Solid Edge part; units mm, degrees
sketch "Sketch1" plane through (0, 0, 0) normal (0, -1, 0) x (1, 0, 0)
  arc A0 (0, 36) -> (-22.6274, 28) centre (0, 0) ccw
  line L0 (-43, 28) -> (-22.6274, 28)
  line L1 (-43, 18) -> (-43, 28)
  line L2 (-22, 18) -> (-43, 18)
  line L3 (-22, 6) -> (-22, 18)
  line L4 (-18.0278, 6) -> (-22, 6)
  arc A1 (0, 19) -> (-18.0278, 6) centre (0, 0) ccw
  arc A2 (0, 19) -> (18.0278, 6) centre (0, 0) cw
  line L5 (18.0278, 6) -> (22, 6)
  line L6 (22, 6) -> (22, 18)
  line L7 (22, 18) -> (43, 18)
  line L8 (43, 18) -> (43, 28)
  line L9 (43, 28) -> (22.6274, 28)
  arc A3 (0, 36) -> (22.6274, 28) centre (0, 0) cw
extrude "Protrusion1" add sketch "Sketch1" along normal mid plane 36
sketch "Sketch2" plane through (32.8137, 0, 28) normal (0, 0, 1) x (0, 1, 0)
  circle A0 centre (0, 32.8137) radius 43
  circle A1 centre (0, 32.8137) radius 50
extrude "ExtrudedCutout_1" cut sketch "Sketch2" against normal blind 61.9029
hole "Hole_1" at (31, 0, 28) direction (0, 0, -1) diameter 10.5 end up to next
sketch "Sketch3" plane through (32.8137, 0, 28) normal (0, 0, 1) x (0, 1, 0)
  circle A0 centre (0, 1.8137) radius 12
extrude "ExtrudedCutout_2" cut sketch "Sketch3" along normal blind 58.8824
mirror "Mirror1" about plane through (0, 0, 0) normal (1, 0, 0) of "Hole_1", "ExtrudedCutout_2"
hole "Hole_2" at (0, 0, 36) direction (0, 0, -1) diameter 6 depth 10 tip angle 118
hole "Hole_3" at (0, 0, 36) direction (0, 0, -1) diameter 3 end through all
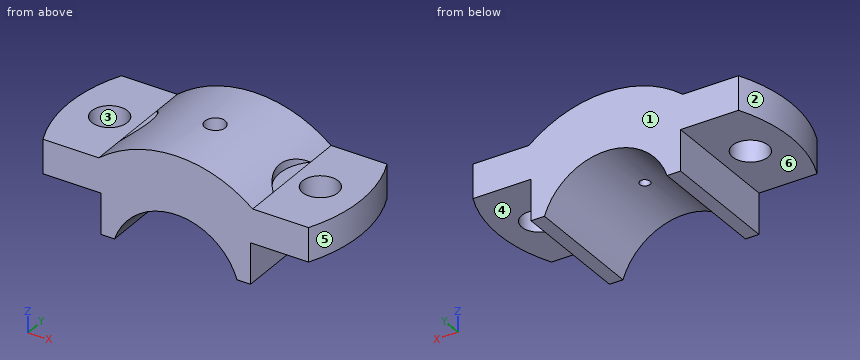
Work out the finished part from the listing and answer in its coordinate system (mm). Face numbers are marked on the shaded views. A direction names the side the tool comes from. Coordinates: 2 decimals unless noted, no trailing zeros. Order: outer loops, then holes, each group sorted by start corner. A loop starts at its lowest first (then second) coordinate and runs counter-clockwise, first axis right, second up. Notation, with made-up numbers: (19, 19.25) - (74, 19.25) arc R29 cw to (74, 48.25) - close; hole circle Ø9 at (55.5, 53). An arc over 180 degrees is marked (long way). Answer as a JSON object with one key per item and string values.
1. Find section B-B on y = 0. Count the separate pieces of the cut face and the enclosed holes in it, plus the area to 3 significant figures.
Output values:
{"separate pieces": "4", "enclosed holes": "0", "area": "990 mm²"}
2. Find section C-C on x = 31. Determine the outline of the cut face in (y, z), plus the area to 3 significant figures.
Output values:
{"outline": "(-18, 18) - (-5.25, 18) - (-5.25, 28) - (-18, 28) - close; (5.25, 18) - (18, 18) - (18, 28) - (5.25, 28) - close", "area": "255 mm²"}
3. The mould has two halves that part along Y. Classify the marked faces 1, 2 and 3: +Y half, -Y half, draft (parallel to the pull), parting line (faces both ways), or undercut.
Output values:
{"face 1": "+Y half", "face 2": "parting line", "face 3": "undercut"}
4. Find section A-A on x = 0. Determine the outline of the cut face in (y, z), plus the area to 3 significant figures.
Output values:
{"outline": "(-18, 19) - (-1.5, 19) - (-1.5, 25.1) - (-3, 26) - (-3, 36) - (-18, 36) - close; (1.5, 19) - (18, 19) - (18, 36) - (3, 36) - (3, 26) - (1.5, 25.1) - close", "area": "530 mm²"}
5. Consider line 1 (X direction, y = 0, z = 22.5); line 2 (Y direction, x = -31, z = 21.75); line 3 (Z direction, x = -37.5, y = -15.5). Determine where each line is inside the solid, lowest interval first.
Output values:
{"line 1": "x = -43 to -36.25, -25.75 to -1.5, 1.5 to 25.75, 36.25 to 43", "line 2": "y = -18 to -5.25, 5.25 to 18", "line 3": "z = 18 to 28"}
6. A tool of negligible diameter and unlimited length cuts with its end or side. For the marked faces 4, 5 and 6, from which of +Z, -Z, +X, -X, +Y, -Y can it reach the whole face along a straight path? Write none if from no direction.
Output values:
{"face 4": "-Z, +X, +Y, -Y", "face 5": "+Z, -Z, +X", "face 6": "-Z, -X, +Y, -Y"}
7. Each of these flat-tipped pins is pushed along its axis until it touches: P1, Ø4, axis at y = 3.5, z = 27, coming from the +X side; P2, Ø6.5, axis at x = -32.5, y = -0.5, coming from the -Z side; P3, Ø12, axis at y = 7.5, z = 20, coming from the -X side; P4, Ø10, axis at x = -36, y = 8.5, coming from the +Z side. Where does it stop, or does it pass through?
Output values:
{"P1": "stops at x = 42.97", "P2": "passes through", "P3": "stops at x = -42.97", "P4": "stops at z = 28"}
8. Find section D-D on z = 13.5. Determine the outline of the cut face in (x, y).
Output values:
{"outline": "(-22, -18) - (-13.37, -18) - (-13.37, 18) - (-22, 18) - close; (13.37, -18) - (22, -18) - (22, 18) - (13.37, 18) - close"}
